```python
from build123d import *

# Parameters (mm, degrees)
RESSALTO_EXTRUS_O1_DEPTH      = 5
RESSALTO_EXTRUS_O2_DEPTH      = 5
RESSALTO_EXTRUS_O3_DEPTH      = 12
RESSALTO_EXTRUS_O3_DEPTH_BACK = 1.993745
ESBO_O4_W                     = 28
ESBO_O4_H                     = 4.585300372


with BuildPart() as part:
    # Esboço1 → Ressalto-extrusão1 (new body)
    with BuildSketch(Plane.XY):
        Polygon((0, 85), (0, 0), (130, 22.922507492), (130, 100.922507492), align=None)
    extrude(amount=RESSALTO_EXTRUS_O1_DEPTH)

    # Esboço3 → Ressalto-extrusão2 (add)
    with BuildSketch(Plane.XY.offset(5)):
        Polygon((-12.113135362, 52.639941774), (0, 54.775814359), (0, 26.775814359), (-12.113135362, 24.639941774), align=None)
    extrude(amount=-RESSALTO_EXTRUS_O2_DEPTH)

    # Esboço4 → Ressalto-extrusão3 (add, two sides: drawn at the far end of the back side and taken through both)
    with BuildSketch(Plane(origin=(-12.015521161, 0, 5.224497292), x_dir=(0, -1, 0), z_dir=(-0.9170600743851252, 0, 0.39874906892524387)).offset(-RESSALTO_EXTRUS_O3_DEPTH_BACK)):
        with Locations((-38.639941774, -2.537451261)):
            Rectangle(ESBO_O4_W, ESBO_O4_H)
    extrude(amount=RESSALTO_EXTRUS_O3_DEPTH + RESSALTO_EXTRUS_O3_DEPTH_BACK)


solid = part.part
```
Source: CAD feature listing. Evaluate the final solid. Frame: model axes, mm. A direction names the side the tool comes from. Round coordinates to 2 decimals unless told otherwise and drop trailing zeros. Loops run counter-clockwise (first coordinate to the right, second up) from the corner with the lowest first, then second, coordinate; pieces in that order, holes last. Notation, with made-up numbers: (14, 11.5) - (73, 11.5) arc R35 cw to (73, 48.5) - close; hole circle Ø8 at (26, -24). An arc over 180 degrees is marked (long way). Use CSV: the item, a comma, the result in double quotes.
Q1. Section query C-C, the plane x = 15. Output: boundary loops of the cut face in (y, z).
Reported:
outline,"(2.64, 0) - (86.84, 0) - (86.84, 5) - (2.64, 5) - close"
Q2. Section query B-B, the plane z = 2.5. Output: boundary loops of the cut face in (x, y).
Reported:
outline,"(-17.86, 24.64) - (-11.03, 24.64) - (-11.03, 24.83) - (0, 26.78) - (0, 0) - (130, 22.92) - (130, 100.92) - (0, 85) - (0, 54.78) - (-12.11, 52.64) - (-17.86, 52.64) - close"
Q3. Section query A-A, the plane y = 31.5. Output: boundary loops of the cut face in (x, z), then the cut area to 3 significant figures.
Reported:
outline,"(-24.95, 5.58) - (-12.11, 0) - (130, 0) - (130, 5) - (-12.11, 5) - (-23.12, 9.78) - close"
area,"770 mm^2"
Q4. Section query D-D, the plane y = 57. Output: boundary loops of the cut face in (x, z).
Reported:
outline,"(0, 0) - (130, 0) - (130, 5) - (0, 5) - close"
Q5. Reachability of faces 1 (the flat face through (130, 61, 2)), 2 (the flat face through (-18, 52.64, 5)), 3 (the flat face through (-18, 24.64, 5)), 4 (the flat face through (58, 51, 5)) from +Z, -Z, +X, -X, +Y, -Y: full face, straight path, thin tool, end or side. Return the list, or none.
Reported:
face 1,"+Z, -Z, +X, +Y, -Y"
face 2,"+Z, -Z, -X, +Y"
face 3,"+Z, -Z, -X, -Y"
face 4,"+Z, +X, +Y, -Y"
Q6. Pin query (flat end, axial travel): pin 1 Ø3 at (x, z) = (-19.5, 7) entering from -Y; pin 2 Ø5 at (x, z) = (21.5, 3) entering from +Y; pin 3 Ø2 at (x, y) = (36, 42.5) entering from +Z; pin 4 Ø6 at (x, y) = (61.5, 39) entering from -Z. Return the tip coordinate at first contact, or that it passes through.
Reported:
pin 1,"y = 24.64"
pin 2,"y = 87.94"
pin 3,"z = 5"
pin 4,"z = 0"
Q7. Ray query, line 1 along X through (y, z) = (75, 3); line 2 along Z through (x, y) = (38.5, 61.5); line 3 along Y through (x, z) = (72, 2.75). Return the intervals inside material, ascending.
Reported:
line 1,"0 to 130"
line 2,"0 to 5"
line 3,"12.7 to 93.82"
